Autodesk Inventor part; units mm, degrees
ref_plane "YZ Plane" through (0, 0, 0) normal (1, 0, 0) x (0, 1, 0)
ref_plane "XZ Plane" through (0, 0, 0) normal (0, 1, 0) x (-1, 0, 0)
ref_plane "XY Plane" through (0, 0, 0) normal (0, 0, 1) x (1, 0, 0)
sketch "Sketch1" plane through (0, 0, 0) normal (0, 0, 1) x (1, 0, 0)
  line L0 (-27.5, 25) -> (27.5, 25)
  line L1 (27.5, 25) -> (27.5, -25)
  line L2 (27.5, -25) -> (-27.5, -25)
  line L3 (-27.5, -25) -> (-27.5, 25)
  line L4 (-27.5, 25) -> (27.5, -25) construction
  line L5 (27.5, 25) -> (-27.5, -25) construction
  point P0 (0, 0)
  dimension "d0" = 55
  dimension "d1" = 50
extrude "Extrusion1" add sketch "Sketch1" along normal blind 6
sketch "Sketch2" plane through (27.5, -25, 0) normal (1, 0, 0) x (0, 0, -1)
  line L0 (-6, 50) -> (-6, 0)
  line L1 (-6, 0) -> (9, 0)
  line L2 (9, 0) -> (9, 50)
  line L3 (9, 50) -> (-6, 50)
  line L4 (-6, 50) -> (-6, 0)
  point P0 (0, 25)
  dimension "d4" = 15
  dimension "d5" = 50
extrude "Extrusion2" add sketch "Sketch2" along normal blind 6
sketch "Sketch4" plane through (27.5, -25, -9) normal (0, 0, -1) x (-1, 0, 0)
  line L0 (0, 0) -> (0, 50)
  line L1 (0, 0) -> (-26, 0)
  line L2 (-26, 0) -> (-26, 50)
  line L3 (-26, 50) -> (0, 50)
  line L4 (0, 50) -> (0, 0)
  point P0 (27.5, 25)
  dimension "d8" = 26
  dimension "d35" = 50
extrude "Extrusion3" add sketch "Sketch4" along normal blind 6
sketch "Sketch5" plane through (27.5, -25, -15) normal (0, 0, -1) x (-1, 0, 0)
  line L0 (0, 50) -> (-26, 50)
  line L1 (-6, 0) -> (-26, 0)
  line L2 (0, 50) -> (-6, 50)
  line L3 (-6, 50) -> (-6, 0)
  line L4 (-6, 0) -> (0, 0)
  line L5 (0, 0) -> (0, 50)
  point P0 (27.5, 25)
  dimension "d11" = 6
extrude "Extrusion4" add sketch "Sketch5" along normal blind 20
sketch "Sketch6" plane through (27.5, -25, -15) normal (0, 0, -1) x (-1, 0, 0)
  line L0 (-6, 0) -> (-26, 0)
  line L1 (-26, 50) -> (-6, 50)
  line L2 (-19, 0) -> (-13, 0)
  line L3 (-13, 0) -> (-13, 50)
  line L4 (-13, 50) -> (-19, 50)
  line L5 (-19, 50) -> (-19, 0)
  line L6 (-26, 50) -> (-26, 0)
  point P0 (27.5, 25)
  dimension "d14" = 6
  dimension "d15" = 7
extrude "Extrusion5" add sketch "Sketch6" along normal blind 1.5 contours L0 L5 L1 L3
sketch "Sketch7" plane through (33.5, -25, -15) normal (1, 0, 0) x (0, 0, -1)
  line L0 (13, 4) -> (7, 4)
  line L1 (7, 4) -> (7, 50)
  line L2 (7, 50) -> (13, 50)
  line L3 (13, 50) -> (13, 4)
  line L4 (20, 50) -> (20, 0)
  line L5 (0, 50) -> (20, 50)
  point P0 (-15, 25)
  dimension "d18" = 6
  dimension "d19" = 46
  dimension "d20" = 7
  dimension "d36" = 0
extrude "Extrusion6" add sketch "Sketch7" along normal blind 1.5
sketch "Sketch8" plane through (27.5, -25, -16.5) normal (0, 0, -1) x (-1, 0, 0)
  line L0 (-13, 0) -> (-13, 50)
  line L1 (-13, 25) -> (-18.895, 25)
  line L2 (-19, 0) -> (-13, 0)
  point P0 (27.5, 25)
  point P1 (-16, 10.5)
  point P2 (-16, 39.5)
  dimension "d23" = 10.5
  dimension "d24" = 3
hole "Hole1" at (43.5, -14.5, -16.5) at (43.5, 14.5, -16.5) direction (0, 0, 1) diameter 6 end through all counterbore diameter 10 counterbore depth 1.5
sketch "Sketch9" plane through (-27.5, -25, 0) normal (0, -1, 0) x (1, 0, 0)
  line L0 (61, -9) -> (61, 6)
  line L1 (0, 6) -> (61, 6)
  line L2 (61, 6) -> (0, 6)
  line L3 (0, 6) -> (0, 0)
  line L4 (0, 0) -> (54.9849, -35)
  line L5 (55, -35) -> (61, -35)
  line L6 (54.9849, -35) -> (61, -35)
  line L7 (61, -35) -> (61, 6)
  point P0 (27.5, 0)
extrude "Extrusion7" add sketch "Sketch9" against normal blind 3
ref_plane "Work Plane1" through (-27.5, 0, 6) normal (0, 1, 0) x (1, 0, 0)
mirror "Mirror1" about plane through (-27.5, 0, 6) normal (0, 1, 0) of "Extrusion7"
ref_plane "Work Plane2" through (43.5, -25, 0) normal (1, 0, 0) x (0, 0, -1)
ref_plane "Work Plane3" through (25, -25, 0) normal (1, 0, 0) x (0, 0, -1)
sketch "Sketch11" plane through (27.5, -25, -35) normal (0, 0, -1) x (-1, 0, 0)
  line L0 (0, 3) -> (0, 47)
  line L1 (0, 3) -> (-3, 3)
  line L2 (-3, 3) -> (-3, 47)
  line L3 (-3, 47) -> (0, 47)
  line L4 (0, 47) -> (0, 3)
  point P0 (27.5, 25)
  point P1 (0, 50)
  dimension "d39" = 3
  dimension "d40" = 44
extrude "Extrusion8" cut sketch "Sketch11" against normal blind 35
sketch "Sketch12" plane through (0, 0, 6) normal (0, 0, 1) x (1, 0, 0)
  arc A0 (15, 17.25) -> (15, 13.75) centre (15, 15.5) ccw
  arc A1 (25, 13.75) -> (25, 17.25) centre (25, 15.5) ccw
  line L0 (-27.5, -22) -> (-27.5, 22)
  line L1 (-27.5, 0) -> (33.5, 0)
  line L2 (33.5, 25) -> (33.5, -25)
  line L3 (-27.5, 25) -> (27.4849, 25)
  line L4 (15, 17.25) -> (25, 17.25)
  line L5 (15, 13.75) -> (25, 13.75)
  line L6 (-27.5, -25) -> (33.5, -25)
  line L7 (-27.5, 25) -> (33.5, 25)
  line L8 (25, 25) -> (25, 0)
  line L9 (25, 16) -> (29.2976, 16)
  line L10 (4.5, 25) -> (4.5, 0)
  arc A2 (-6, 13.75) -> (-6, 17.25) centre (-6, 15.5) ccw
  arc A3 (-16, 17.25) -> (-16, 13.75) centre (-16, 15.5) ccw
  line L11 (-6, 17.25) -> (-16, 17.25)
  line L12 (-6, 13.75) -> (-16, 13.75)
  arc A4 (15, -13.75) -> (15, -17.25) centre (15, -15.5) ccw
  arc A5 (25, -17.25) -> (25, -13.75) centre (25, -15.5) ccw
  line L13 (15, -17.25) -> (25, -17.25)
  line L14 (15, -13.75) -> (25, -13.75)
  arc A6 (-16, -13.75) -> (-16, -17.25) centre (-16, -15.5) ccw
  line L15 (-6, -17.25) -> (-16, -17.25)
  line L16 (-6, -13.75) -> (-16, -13.75)
  arc A7 (-6, -17.25) -> (-6, -13.75) centre (-6, -15.5) ccw
  arc A8 (-0.5, 11.5) -> (-0.5, -11.5) centre (-0.5, 0) ccw
  arc A9 (9.5, -11.5) -> (9.5, 11.5) centre (9.5, 0) ccw
  line L17 (-0.5, 11.5) -> (9.5, 11.5)
  line L18 (9.5, -11.5) -> (-0.5, -11.5)
  point P0 (0, 0)
  point P1 (-16, 16)
  point P2 (25, -16)
  point P3 (-16, -16)
  point P4 (33.5, 29)
  dimension "d43" = 3.5
  dimension "d44" = 3.5
  dimension "d49" = 8.5
  dimension "d51" = 20.5
  dimension "d52" = 15.5
  dimension "d53" = 23
  dimension "d54" = 23
  dimension "d55" = 5
  dimension "d56" = 5
extrude "Extrusion9" cut sketch "Sketch12" against normal blind 42 contours L4 L8 L5 A0 | A1 L9 L8 | L8 L9 A1 | A9 L18 A8 L1 | L1 L10 L17 A9 | L10 L1 A8 L17 | L12 A3 L11 A2 | L14 A5 L13 A4 | L16 A7 L15 A6
sketch "Sketch14" plane through (0, 0, 6) normal (0, 0, 1) x (1, 0, 0)
  arc A0 (-16, 17.25) -> (-16, 13.75) centre (-16, 15.5) ccw
  arc A1 (-16, 19.5) -> (-16, 11.5) centre (-16, 15.5) ccw
  arc A2 (-6, 13.75) -> (-6, 17.25) centre (-6, 15.5) ccw
  arc A3 (-6, 11.5) -> (-6, 19.5) centre (-6, 15.5) ccw
  line L0 (-16, 19.5) -> (-6, 19.5)
  line L1 (-6, 11.5) -> (-16, 11.5)
  arc A4 (15, 17.25) -> (15, 13.75) centre (15, 15.5) ccw
  arc A5 (15, -13.75) -> (15, -17.25) centre (15, -15.5) ccw
  arc A6 (-16, -13.75) -> (-16, -17.25) centre (-16, -15.5) ccw
  arc A7 (15, 19.5) -> (15, 11.5) centre (15, 15.5) ccw
  arc A8 (25, 11.5) -> (25, 19.5) centre (25, 15.5) ccw
  line L2 (15, 19.5) -> (25, 19.5)
  line L3 (25, 11.5) -> (15, 11.5)
  arc A9 (15, -11.5) -> (15, -19.5) centre (15, -15.5) ccw
  arc A10 (25, -19.5) -> (25, -11.5) centre (25, -15.5) ccw
  line L4 (15, -11.5) -> (25, -11.5)
  line L5 (25, -19.5) -> (15, -19.5)
  arc A11 (-16, -11.5) -> (-16, -19.5) centre (-16, -15.5) ccw
  arc A12 (-6, -19.5) -> (-6, -11.5) centre (-6, -15.5) ccw
  line L6 (-16, -11.5) -> (-6, -11.5)
  line L7 (-6, -19.5) -> (-16, -19.5)
  point P0 (0, 0)
  dimension "d59" = 8
  dimension "d60" = 8
  dimension "d61" = 8
  dimension "d62" = 8
  dimension "d63" = 8
  dimension "d64" = 8
  dimension "d65" = 8
  dimension "d66" = 8
extrude "Extrusion10" cut sketch "Sketch14" against normal blind 3
chamfer "Chamfer1" distance 3 angle 45 1 edges at (33.5, 0, -9)
fillet "Fillet1" radius 2 6 edges at (-27.5, -25, 3) (-27.5, 25, 3) (-27.5, 0, 6) (53.5, 25, -12) (53.5, -25, -12) (53.5, 0, -9)
properties part number "Estrutura - Suporte Z Motor v2"
Input: part model. Units: mm. Frame: model coordinates. A direction names the side the tool comes from. Round coordinates to 2 decimals unless told otherwise and drop trailing zeros. Loops run counter-clockwise (first coordinate to the right, second up) from the corner with the lowest first, then second, coordinate; pieces in that order, holes last.
1) Section query C-C on x = 7. Return the cut outline in (y, z), plus the area to 3 significant figures.
Ans:
outline: (-25, -21.96) - (-22, -21.96) - (-22, 0) - (-11.5, 0) - (-11.5, 6) - (-25, 6) - close; (11.5, 0) - (22, 0) - (22, -21.96) - (25, -21.96) - (25, 6) - (11.5, 6) - close
area: 294 mm2
2) Section query D-D on z = -7.5. Return the cut outline in (x, y), plus the area to 3 significant figures.
Ans:
outline: (-15.72, -25) - (35, -25) - (35, 25) - (-15.72, 25) - (-15.72, 22) - (30.5, 22) - (30.5, -22) - (-15.72, -22) - close
area: 502 mm2
3) Set-up query: faces 5 (the cylindrical face through (-20, -15.4, 4.5)), 6 (the flat face through (44, 22, -16.5)), 7 (the cylindrical face through (-4.25, 15.46, 1.52)). Return all of +Z, -Z, +X, -X, +Y, -Y with unobstructed straight access to the full face (end or side cutting, diameter ignored); none if empty.
Ans:
face 5: +Z
face 6: -Z, +X, +Y, -Y
face 7: +Z, -Z
4) Section query B-B on y = 0. Return the cut outline in (x, z).
Ans:
outline: (-27.5, 0) - (-12, 0) - (-12, 6) - (-25.5, 6) arc R2 ccw to (-27.5, 4) - close; (21, 0) - (30.5, 0) - (30.5, -35) - (33.5, -35) - (33.5, -28) - (35, -28) - (35, -22) - (33.5, -22) - (33.5, -15) - (40.5, -15) - (40.5, -16.5) - (46.5, -16.5) - (46.5, -15) - (53.5, -15) - (53.5, -11) arc R2 ccw to (51.5, -9) - (36.5, -9) - (33.5, -6) - (33.5, 6) - (21, 6) - close
5) Section query A-A on x = 43.5. Return the cut outline in (y, z).
Ans:
outline: (-25, -16.5) - (-19.5, -16.5) - (-19.5, -15) - (-17.5, -15) - (-17.5, -9) - (-25, -9) - close; (-11.5, -15) - (-9.5, -15) - (-9.5, -16.5) - (9.5, -16.5) - (9.5, -15) - (11.5, -15) - (11.5, -9) - (-11.5, -9) - close; (17.5, -15) - (19.5, -15) - (19.5, -16.5) - (25, -16.5) - (25, -9) - (17.5, -9) - close
6) Material intervals for line 1 (Y direction, x = 43.5, z = -12.2); line 2 (Y direction, x = 14.5, z = -4.5); line 3 (X direction, y = -14.5, z = 0.5), sorted ascending.
Ans:
line 1: y = -25 to -17.5, -11.5 to 11.5, 17.5 to 25
line 2: y = -25 to -22, 22 to 25
line 3: x = -27.5 to -17.44, -4.56 to 13.56, 26.44 to 33.5
7) Pin query (flat end, axial travel): pin 1 (2 mm diameter, centred on y = 9.5, z = -26.5, fed in from -X); pin 2 (2.5 mm diameter, centred on x = -12, y = -14.5, fed in from +Z); pin 3 (7 mm diameter, centred on x = 43.5, y = 14.5, fed in from -Z). Return the tip coordinate at first contact, or that it passes through.
Ans:
pin 1: stops at x = 30.5
pin 2: stops at z = 3
pin 3: stops at z = -15
8) Pull-direction query (X, two-part tool) for faces 1 (the flat face through (-11, 18, 3)), 2 (the cylindrical face through (-26.9, 24.43, 2.41)), 3 (the flat face through (-11, 19.5, 5)), 4 (the flat face through (44, 0, -16.5)); classes: released by +X, released by -X, zero draft, split by the parting line, or undercut.
Ans:
face 1: undercut
face 2: released by -X
face 3: undercut
face 4: zero draft
